Part print with two shaded views. Sizes in mm from the minimum x, y, z corner. A direction names the side the tool comes from. Give positions to 0.01 mm unless a question says otherwise; leave off trailing zeros. Write each loop counter-clockwise with the first axis right and the second up, starting at its lowest first coordinate (ties: lowest second). Pieces come first, ordered by that corner, then holes. Notation, with made-up numbers: (-10.75, -19) - (28.25, -19) arc R16 cw to (28.25, -1) - close; hole circle Ø4 at (54.25, 9.5). An arc over 180 degrees is marked (long way). Answer as a JSON object with one key per item and string values.
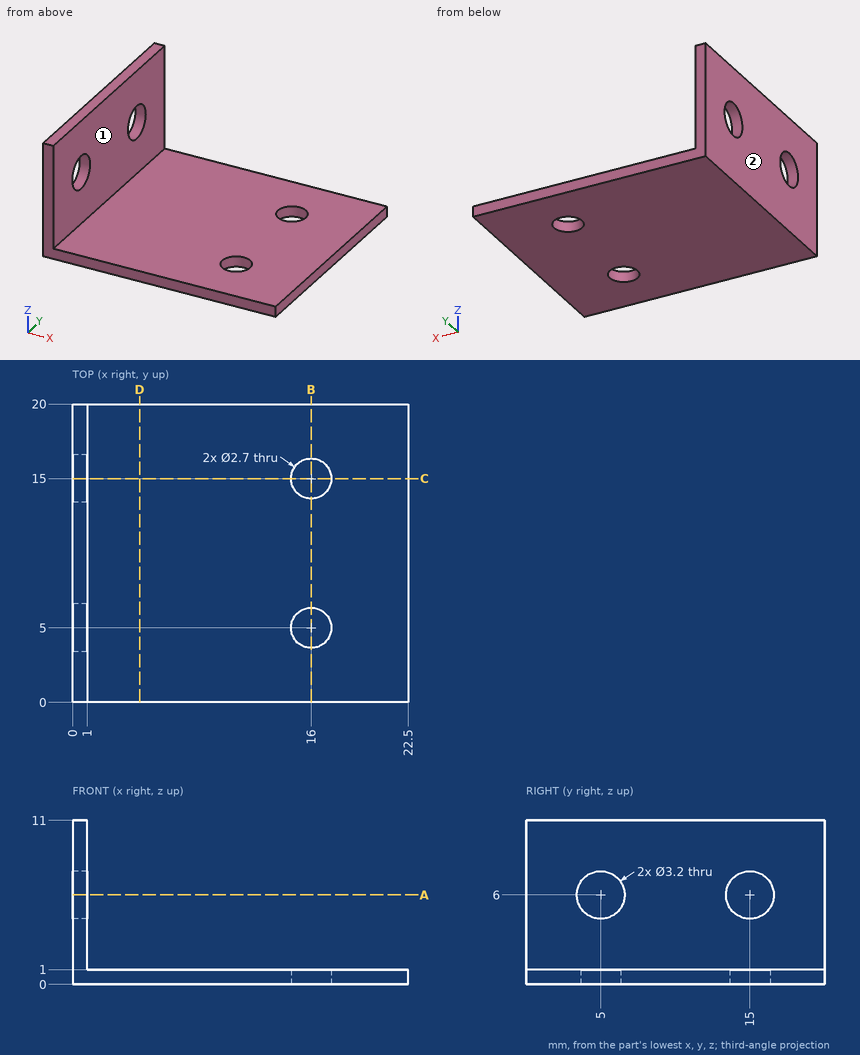
(1) Probe L1, parallel to Y at x = 0.7, z = 6; L2, parallel to Y at x = 16, z = 0.4; L3, parallel to X at y = 15, z = 0.6. List the from-to ranges inside material, lowest first. Write a range as [from, to].
Answer key:
{"L1": "y = [0, 3.4], [6.6, 13.4], [16.6, 20]", "L2": "y = [0, 3.65], [6.35, 13.65], [16.35, 20]", "L3": "x = [0, 14.65], [17.35, 22.5]"}
(2) Saw through at C-C, the plane y = 15. Give the cut face in (x, z).
Answer key:
{"outline": "(0, 0) - (14.65, 0) - (14.65, 1) - (1, 1) - (1, 4.4) - (0, 4.4) - close; (0, 7.6) - (1, 7.6) - (1, 11) - (0, 11) - close; (17.35, 0) - (22.5, 0) - (22.5, 1) - (17.35, 1) - close"}
(3) Flat gauge pins, fed straight in: P1, Ø3, axis at y = 3, z = 6, coming from the +X side; P2, Ø4, axis at y = 15, z = 6, coming from the -X side; P3, Ø4.5, axis at x = 16, y = 15, coming from the +Z side. Where does each tip first touch, or does it go through?
Answer key:
{"P1": "stops at x = 1", "P2": "stops at x = 0", "P3": "stops at z = 1"}
(4) 3-axis set-ups, long thin cutter, end or side, ignore diameter. For the marked faces 1 and 2: which of +Z, -Z, +X, -X, +Y, -Y reach the whole face in a straight line?
Answer key:
{"face 1": "+Z, +X, +Y, -Y", "face 2": "+Z, -Z, -X, +Y, -Y"}
(5) Saw through at A-A, the plane z = 6. Give the cut face in (x, y), and give its area (3 significant figures).
Answer key:
{"outline": "(0, 0) - (1, 0) - (1, 3.4) - (0, 3.4) - close; (0, 6.6) - (1, 6.6) - (1, 13.4) - (0, 13.4) - close; (0, 16.6) - (1, 16.6) - (1, 20) - (0, 20) - close", "area": "13.6 mm²"}
(6) Saw through at D-D, the plane x = 4.5. Give the cut face in (y, z), and give its area (3 significant figures).
Answer key:
{"outline": "(0, 0) - (20, 0) - (20, 1) - (0, 1) - close", "area": "20.0 mm²"}
(7) Saw through at B-B, the plane x = 16. Give the cut face in (y, z).
Answer key:
{"outline": "(0, 0) - (3.65, 0) - (3.65, 1) - (0, 1) - close; (6.35, 0) - (13.65, 0) - (13.65, 1) - (6.35, 1) - close; (16.35, 0) - (20, 0) - (20, 1) - (16.35, 1) - close"}
